Source: CAD feature listing. Evaluate the final solid. Frame: model axes, mm. Round coordinates to 2 decimals unless told otherwise and drop trailing zeros. Write each loop counter-clockwise with the first axis right and the second up, starting at its lowest first coordinate (ties: lowest second). Pieces come first, ordered by that corner, then holes. Notation, with made-up numbers: (-5.5, -28) -> (15.5, -28) arc R18 ccw to (15.5, -7) -> close; hole circle Ø6 at (46.25, -35). An arc over 180 degrees is marked (long way). Put each result on its own line as item: value.
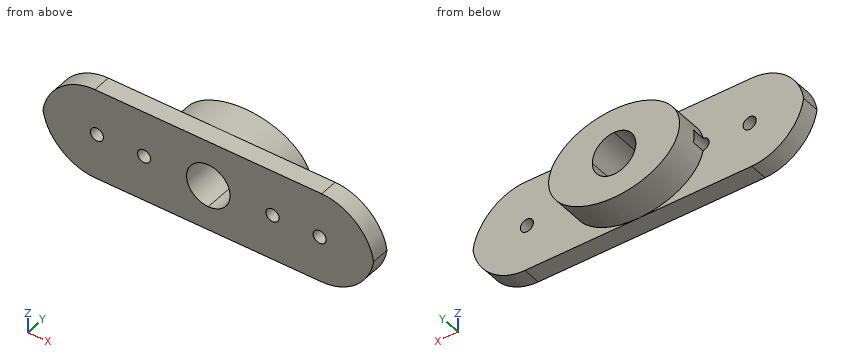
```python
from build123d import *

# Parameters (mm, degrees)
SKETCH1_W               = 32.1564
SKETCH1_H               = 8.89
SKETCH1_R               = 1.2319
BOSS_EXTRUDE1_DEPTH     = 1.778
CUT_EXTRUDE1_DEPTH      = 32.409990197
CUT_EXTRUDE1_DEPTH_BACK = 34.409990197
CUT_EXTRUDE1_START      = 2
FILLET1_SIZE            = 5.08
SKETCH1_7_RX            = 6.35
SKETCH1_7_RY            = 4.445
BOSS_EXTRUDE2_DEPTH     = 5
CUT_EXTRUDE2_DEPTH      = 34.69313211
CUT_EXTRUDE2_DEPTH_BACK = 34.69313211
CUT_EXTRUDE3_DEPTH      = 1.27
CUT_EXTRUDE3_DEPTH_BACK = 12.7
SKETCH2_R               = 0.635


with BuildPart() as part:
    # Sketch1 → Boss-Extrude1 (new body)
    with BuildSketch(Plane(origin=(0, 0, 0), x_dir=(1, 0, 0), z_dir=(0, 1, 0))):
        with Locations((16.0782, 4.445)):
            Rectangle(SKETCH1_W, SKETCH1_H)
        with Locations(Location((16.0782, 4.445, 0), (0, 0, 270))):
            Circle(SKETCH1_R, mode=Mode.SUBTRACT)
    extrude(amount=BOSS_EXTRUDE1_DEPTH)

    # Sketch1<5> → Cut-Extrude1 (cut, two sides: drawn at the far end of the back side and taken through both)
    with BuildSketch(Plane(origin=(0, 0, 0), x_dir=(1, 0, 0), z_dir=(0, 1, 0)).offset(CUT_EXTRUDE1_START - CUT_EXTRUDE1_DEPTH_BACK)):
        with BuildLine():
            ThreePointArc((18.1864, 4.445), (17.568922516, 5.935722516), (16.0782, 6.5532))
            Line((16.0782, 6.5532), (16.0782, 5.6769))
            ThreePointArc((16.0782, 5.6769), (16.949284844, 5.316084844), (17.3101, 4.445))
            ThreePointArc((17.3101, 4.445), (16.949284844, 3.573915156), (16.0782, 3.2131))
            Line((16.0782, 3.2131), (16.0782, 2.3368))
            ThreePointArc((16.0782, 2.3368), (17.568922516, 2.954277484), (18.1864, 4.445))
        make_face()
        with BuildLine():
            Line((16.0782, 5.6769), (16.0782, 6.5532))
            ThreePointArc((16.0782, 6.5532), (13.97, 4.445), (16.0782, 2.3368))
            Line((16.0782, 2.3368), (16.0782, 3.2131))
            ThreePointArc((16.0782, 3.2131), (14.8463, 4.445), (16.0782, 5.6769))
        make_face()
        with BuildLine():
            ThreePointArc((17.3101, 4.445), (16.949284844, 5.316084844), (16.0782, 5.6769))
            Line((16.0782, 5.6769), (16.0782, 3.2131))
            ThreePointArc((16.0782, 3.2131), (16.949284844, 3.573915156), (17.3101, 4.445))
        make_face()
        with BuildLine():
            Line((16.0782, 3.2131), (16.0782, 5.6769))
            ThreePointArc((16.0782, 5.6769), (14.8463, 4.445), (16.0782, 3.2131))
        make_face()
    extrude(amount=CUT_EXTRUDE1_DEPTH + CUT_EXTRUDE1_DEPTH_BACK, mode=Mode.SUBTRACT)

    # Fillet1
    # a fillet whose section is not a circle: 5.08 mm, written as the material it takes off along each edge
    with BuildSketch(Plane(origin=(32.1564, -12.7, -8.89), x_dir=(0, 0, 1), z_dir=(0, 1, 0)), Plane(origin=(32.1564, -12.7, 0), x_dir=(-1, 0, 0), z_dir=(0, 1, 0))) as fillet1_piece_1:
        with BuildLine():
            Bezier((FILLET1_SIZE, 0), (0, 0), (0, -FILLET1_SIZE), weights=[1, 0.666666667, 1])
            Line((0, -FILLET1_SIZE), (0, 0))
            Line((0, 0), (FILLET1_SIZE, 0))
        make_face()
    extrude(amount=27.178, mode=Mode.SUBTRACT)
    with BuildSketch(Plane(origin=(0, -12.7, -8.89), x_dir=(0, 0, 1), z_dir=(0, 1, 0)), Plane(origin=(0, -12.7, 0), x_dir=(1, 0, 0), z_dir=(0, 1, 0))) as fillet1_piece_2:
        with BuildLine():
            Bezier((FILLET1_SIZE, 0), (0, 0), (0, FILLET1_SIZE), weights=[1, 0.666666667, 1])
            Line((0, FILLET1_SIZE), (0, 0))
            Line((0, 0), (FILLET1_SIZE, 0))
        make_face()
    extrude(amount=27.178, mode=Mode.SUBTRACT)

    # Sketch1<7> → Boss-Extrude2 (add)
    with BuildSketch(Plane(origin=(0, 0, 0), x_dir=(1, 0, 0), z_dir=(0, 1, 0))):
        with Locations(Location((16.0782, 4.445), (0, 0, 0))):
            Ellipse(SKETCH1_7_RX, SKETCH1_7_RY)
    extrude(amount=BOSS_EXTRUDE2_DEPTH)

    # Sketch1<8> → Cut-Extrude2 (cut, two sides: drawn at the far end of the back side and taken through both)
    with BuildSketch(Plane(origin=(0, 0, 0), x_dir=(1, 0, 0), z_dir=(0, 1, 0)).offset(-CUT_EXTRUDE2_DEPTH_BACK)):
        with BuildLine():
            ThreePointArc((18.1864, 4.445), (17.568922516, 5.935722516), (16.0782, 6.5532))
            Line((16.0782, 6.5532), (16.0782, 5.6769))
            ThreePointArc((16.0782, 5.6769), (16.949284844, 5.316084844), (17.3101, 4.445))
            ThreePointArc((17.3101, 4.445), (16.949284844, 3.573915156), (16.0782, 3.2131))
            Line((16.0782, 3.2131), (16.0782, 2.3368))
            ThreePointArc((16.0782, 2.3368), (17.568922516, 2.954277484), (18.1864, 4.445))
        make_face()
        with BuildLine():
            Line((16.0782, 5.6769), (16.0782, 6.5532))
            ThreePointArc((16.0782, 6.5532), (13.97, 4.445), (16.0782, 2.3368))
            Line((16.0782, 2.3368), (16.0782, 3.2131))
            ThreePointArc((16.0782, 3.2131), (14.8463, 4.445), (16.0782, 5.6769))
        make_face()
    extrude(amount=CUT_EXTRUDE2_DEPTH + CUT_EXTRUDE2_DEPTH_BACK, mode=Mode.SUBTRACT)


with BuildPart() as cut_extrude2_kept_piece:
    # of the separate pieces the step leaves, the one the design keeps (cut_extrude2_pieces_kept)
    add(part.part.solids().sort_by_distance((5.08, 0, 0))[0])

    # Sketch2 → Cut-Extrude3 (cut, two sides: drawn at the far end of the back side and taken through both)
    with BuildSketch(Plane(origin=(0, 1.778, 0), x_dir=(1, 0, 0), z_dir=(0, 1, 0)).offset(-CUT_EXTRUDE3_DEPTH_BACK)):
        with Locations(Location((9.848128616, 4.444938826, 0), (0, 0, 94.99673829))):
            Circle(SKETCH2_R)
        with Locations(Location((5.276128616, 4.444938826, 0), (0, 0, 270))):
            Circle(SKETCH2_R)
        with Locations(Location((22.308288089, 4.444938826, 0), (0, 0, 85.004802362))):
            Circle(SKETCH2_R)
        with Locations(Location((26.880288089, 4.444938826, 0), (0, 0, 270))):
            Circle(SKETCH2_R)
    extrude(amount=CUT_EXTRUDE3_DEPTH + CUT_EXTRUDE3_DEPTH_BACK, mode=Mode.SUBTRACT)


solid = cut_extrude2_kept_piece.part
```
Q1. Cut plane A-A on x = 25. Output: boundary loops of the cut face in (y, z), and give its area (3 significant figures).
Ans:
outline: (0, -8.89) -> (1.78, -8.89) -> (1.78, 0) -> (0, 0) -> close
area: 15.8 mm^2
Q2. Pin query (flat end, axial travel): pin 1 (1 mm diameter, centred on x = 22.31, z = -4.44, fed in from -Y); pin 2 (1.7 mm diameter, centred on x = 9.85, z = -4.44, fed in from -Y); pin 3 (1 mm diameter, centred on y = 3, z = -3.5, fed in from +X). Return the tip coordinate at first contact, or that it passes through.
Ans:
pin 1: stops at y = 3.05
pin 2: stops at y = 0
pin 3: stops at x = 22.4
Q3. Material intervals for line 1 (X direction, y = 1.2, z = -5); line 2 (Z direction, x = 17, y = 2); line 3 (X direction, y = 2.55, z = -3), sorted ascending. Write a range as [from, to].
Ans:
line 1: x = [0.15, 4.97], [5.58, 9.54], [10.16, 14.04], [18.11, 22], [22.62, 26.57], [27.19, 32]
line 2: z = [-8.84, -6.34], [-2.55, -0.05]
line 3: x = [10.07, 14.54], [17.61, 22.08]
Q4. Cut plane B-B on y = 0.85. Give the number of separate pieces and of enclosed holes in the cut face, and give its area (3 significant figures).
Ans:
separate pieces: 1
enclosed holes: 5
area: 244 mm^2
